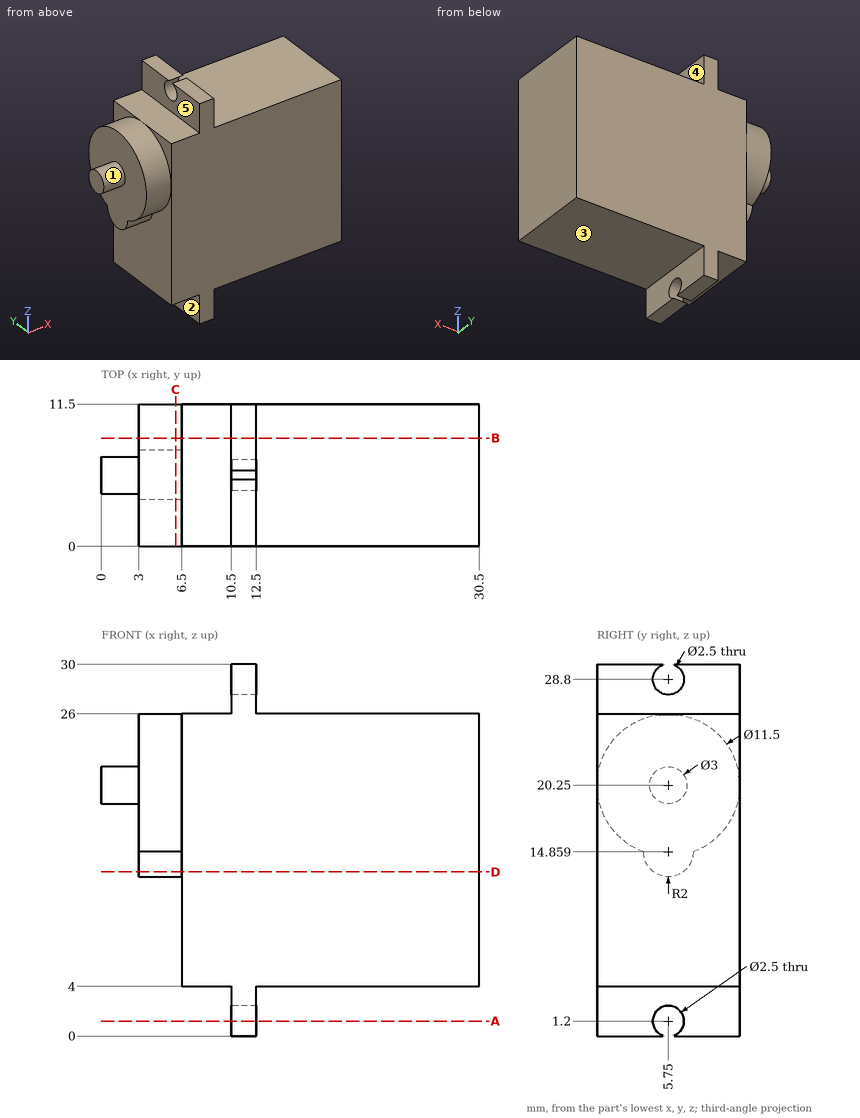
Could you check a few things on this drawing? It's one solid part, dimensions in mm from its lowest x, y, z. A direction names the side the tool comes from. Coordinates: 2 decimals unless noted, no trailing zeros. Order: outer loops, then holes, each group sorted by start corner. A loop starts at its lowest first (then second) coordinate and runs counter-clockwise, first axis right, second up. Notation, with made-up numbers: (87, 48) - (137, 48) arc R35 ccw to (137, 86) - close; hole circle Ø8 at (63.25, 66.25). An arc over 180 degrees is marked (long way). Answer as a JSON object with one key per item and string values. Group by question number.
Q1. Imagine slicing it at B-B (y = 8.75). Please give me the cut outline in (x, z), and give its area (3 significant figures).
Q2. Imagine slicing it at D-D (z = 13.25). Please give me the cut outline in (x, y).
Q3. On a 3-axis mill with a long thin cutter (end or side, diameter ignored), from which of +Z, -Z, +X, -X, +Y, -Y can I reach the whole of each face in a straight line? I mean the marked faces 1, 2, 3, 4 and 5. Say none if no direction works.
Q4. Will these pins go through, and if not, where does the flat tip stop? P1, Ø6, axis at x = 21, y = 3.5, coming from the -Z side; P2, Ø4.5, axis at y = 7.5, z = 2.5, coming from the -X side; P3, Ø4.5, axis at y = 5, z = 27, coming from the -X side.
Q5. Imagine slicing it at C-C (x = 6). Please give me the cut outline in (y, z), and give its area (3 significant figures).
Q6. Imagine slicing it at A-A (z = 1.2). Please give me the cut outline in (x, y).
Q7. I need wall thicknesses on line 1 (Y direction, x = 11.1, z = 1.2); line 2 (X direction, y = 5.25, z = 3.75); line 3 (Z direction, x = 29.5, y = 7.5). Which ranges of each line are inside material? Lowest first, please. Write a range as from..to.
Determined:
{
 "1": {"outline": "(3, 15.34) - (6.5, 15.34) - (6.5, 4) - (10.5, 4) - (10.5, 0) - (12.5, 0) - (12.5, 4) - (30.5, 4) - (30.5, 26) - (12.5, 26) - (12.5, 30) - (10.5, 30) - (10.5, 26) - (6.5, 26) - (6.5, 25.16) - (3, 25.16) - close", "area": "578 mm2"},
 "2": {"outline": "(3, 4.56) - (6.5, 4.56) - (6.5, 0) - (30.5, 0) - (30.5, 11.5) - (6.5, 11.5) - (6.5, 6.94) - (3, 6.94) - close"},
 "3": {"face 1": "-X", "face 2": "-Z, -X, +Y, -Y", "face 3": "-Z, +X, +Y, -Y", "face 4": "+Z, +X, +Y, -Y", "face 5": "+Z, -X, +Y, -Y"},
 "4": {"P1": "stops at z = 4", "P2": "stops at x = 6.5", "P3": "stops at x = 3"},
 "5": {"outline": "(3.75, 14.86) arc R2 ccw to (7.75, 14.86) arc R5.75 ccw (long way) to start", "area": "109 mm2"},
 "6": {"outline": "(10.5, 0) - (12.5, 0) - (12.5, 4.5) - (10.5, 4.5) - close; (10.5, 7) - (12.5, 7) - (12.5, 11.5) - (10.5, 11.5) - close"},
 "7": {"line 1": "y = 0..4.5, 7..11.5", "line 2": "x = 10.5..12.5", "line 3": "z = 4..26"}
}
